Source: CAD feature listing. Evaluate the final solid. Frame: model axes, mm. A direction names the side the tool comes from. Give positions to 0.01 mm unless a question says otherwise; leave off trailing zeros. Loops run counter-clockwise (first coordinate to the right, second up) from the corner with the lowest first, then second, coordinate; pieces in that order, holes last. Notation, with made-up numbers: (6.25, 47.5) -> (42.25, 47.5) arc R13 ccw to (42.25, 60.5) -> close; hole circle Ø4 at (75, 77.25). An arc over 180 degrees is marked (long way). Return JSON: item names as keys, results as strings. Group by question number.
(1) Cut plane C-C on y = 15. Return loops of the section in (x, z).
(2) Pin query (flat end, axial travel): pin 1 (8 mm diameter, centred on x = -1, y = 1.5, fed in from +Z); pin 2 (1.5 mm diameter, centred on x = -6, y = 11.5, fed in from +Z); pin 3 (9 mm diameter, centred on x = 0, y = 0, fed in from -Z); pin 4 (3 mm diameter, centred on x = -1.5, z = 13.5, fed in from -Y). Return the tip coordinate at first contact, or that it passes through.
(3) Draft query along X for faces 4 (the face through (18, 0, 6)), 5 (the face through (-7, -15.429, 5)), 6 (the face through (0, 12.363, 13)). Return one class per face: released by +X, released by -X, zero draft, split by the parting line, or undercut.
(4) Cut plane B-B on z = 4. Give the number of separate pieces and of enclosed holes in the cut face, then the cut area to 3 significant figures.
(5) Cut plane A-A on z = 8.75. Return loops of the section in (x, y).
(6) Cut plane D-D on x = 11. Return loops of the section in (y, z), then the cut area to 3 significant figures.
(7) Access query for faces 1 (the face through (-7, -10.629, 5)), 2 (the face through (-12.363, 0, 13)), 3 (the face through (12.363, 0, 13)). Directions: +Z, -Z, +X, -X, +Y, -Y. A direction counts if a zero-diameter tool reaches every point of the face in a straight line with its end or side. Return the directions, or none.
(8) Ray query, line 1 (Y direction, x = 0, z = 12.3); line 2 (Y direction, x = -10, z = 4.75); line 3 (Z direction, x = -13, y = -13.5). Return the intervals inside material, ascending. Write a range as from..to.
```python
from build123d import *

# Parameters (mm, degrees)
BOSS_EXTRUDE1_DEPTH = 11.868131868
SKETCH2_R           = 1.5
CUT_EXTRUDE1_DEPTH  = 5
BOSS_EXTRUDE2_DEPTH = 2.769230769
SKETCH7_W           = 8.5
SKETCH7_H           = 4.8
SKETCH7_W_2         = 0.5
SKETCH7_H_2         = 0.5
CUT_EXTRUDE2_DEPTH  = 10


with BuildPart() as part:
    # Sketch1 → Boss-Extrude1 (new body)
    with BuildSketch(Plane.XY):
        with BuildLine():
            Line((-16, 18), (16, 18))
            ThreePointArc((16, 18), (17.414213562, 17.414213562), (18, 16))
            Line((18, 16), (18, -16))
            ThreePointArc((18, -16), (17.414213562, -17.414213562), (16, -18))
            Line((16, -18), (-16, -18))
            ThreePointArc((-16, -18), (-17.414213562, -17.414213562), (-18, -16))
            Line((-18, -16), (-18, 16))
            ThreePointArc((-18, 16), (-17.414213562, 17.414213562), (-16, 18))
        make_face()
    extrude(amount=BOSS_EXTRUDE1_DEPTH)

    # Sketch2 → Cut-Extrude1 (cut)
    with BuildSketch(Plane(origin=(0, 0, 0), x_dir=(-1, 0, 0), z_dir=(0, 0, -1))):
        with Locations((-13.554503907, -13.802086098)):
            Circle(SKETCH2_R)
        with Locations((14.445496093, 14.197913902)):
            Circle(SKETCH2_R)
    extrude(amount=-CUT_EXTRUDE1_DEPTH, mode=Mode.SUBTRACT)

    # Sketch3 → Boss-Extrude2 (add)
    with BuildSketch(Plane.XY.offset(11.868131868)):
        with BuildLine():
            Line((-10.362637363, 12.362637363), (10.362637363, 12.362637363))
            ThreePointArc((10.362637363, 12.362637363), (11.776850925, 11.776850925), (12.362637363, 10.362637363))
            Line((12.362637363, 10.362637363), (12.362637363, -10.362637363))
            ThreePointArc((12.362637363, -10.362637363), (11.776850925, -11.776850925), (10.362637363, -12.362637363))
            Line((10.362637363, -12.362637363), (-10.362637363, -12.362637363))
            ThreePointArc((-10.362637363, -12.362637363), (-11.776850925, -11.776850925), (-12.362637363, -10.362637363))
            Line((-12.362637363, -10.362637363), (-12.362637363, 10.362637363))
            ThreePointArc((-12.362637363, 10.362637363), (-11.776850925, 11.776850925), (-10.362637363, 12.362637363))
        make_face()
    extrude(amount=BOSS_EXTRUDE2_DEPTH)

    # Sketch4 → Revolve1 (revolve)
    with BuildSketch(Plane(origin=(0, 0, 0), x_dir=(1, 0, 0), z_dir=(0, 1, 0)), mode=Mode.PRIVATE) as revolve1_sk:
        Polygon((-8.33139296, -14.637362637), (-8.202720326, -14.837362637), (-8.040760547, -14.837362637), (-7.912087912, -14.637362637), align=None)
    revolve(revolve1_sk.sketch.rotate(Axis((0, 0, 15.476177455), (0, 0, 1)), 180), axis=Axis((0, 0, 15.476177455), (0, 0, 1)))

    # Sketch5 → Cut-Revolve1 (revolve, cut)
    with BuildSketch(Plane(origin=(0, 0, 0), x_dir=(1, 0, 0), z_dir=(0, 1, 0)), mode=Mode.PRIVATE) as cut_revolve1_sk:
        Polygon((-7.912087912, -14.637362637), (-5.918480504, -13.782101407), (-5.718480504, -13.782101407), (-5.718480504, -13.582101407), (-5.518480504, -13.582101407), (-5.518480504, -13.382101407), (-5.318480504, -13.382101407), (-5.318480504, -13.182101407), (-5.118480504, -13.182101407), (-5.118480504, -12.982101407), (-4.918480504, -12.982101407), (-4.918480504, -12.782101407), (-4.718480504, -12.782101407), (-4.718480504, -12.582101407), (-4.518480504, -12.582101407), (-4.518480504, -12.382101407), (-4.318480504, -12.382101407), (-4.318480504, -12.182101407), (-4.118480504, -12.182101407), (-4.118480504, -11.982101407), (-3.918480504, -11.982101407), (-3.918480504, -11.782101407), (0, -11.782101407), (0, -14.637362637), align=None)
    revolve(cut_revolve1_sk.sketch.rotate(Axis((0, 0, 19.146341311), (0, 0, -1)), 180), axis=Axis((0, 0, 19.146341311), (0, 0, -1)), mode=Mode.SUBTRACT)

    # Sketch6 → Revolve2 (revolve)
    with BuildSketch(Plane(origin=(0, 0, 0), x_dir=(1, 0, 0), z_dir=(0, 1, 0))):
        with BuildLine():
            Line((-3.308329692, -11.782101407), (-3.308329692, -12.908378043))
            Line((-3.308329692, -12.908378043), (-2.963068503, -12.908378043))
            ThreePointArc((-2.963068503, -12.908378043), (-1.670669607, -14.043416814), (0, -14.452649))
            Line((0, -14.452649), (0, -11.782101407))
            Line((0, -11.782101407), (-3.308329692, -11.782101407))
        make_face()
    revolve(axis=Axis((0, 0, 14.452649), (0, 0, -1)))

    # Sketch7 → Cut-Extrude2 (cut)
    with BuildSketch(Plane(origin=(0, 0, 0), x_dir=(-1, 0, 0), z_dir=(0, 0, -1))):
        with Locations((6.826923077, -13.028571429)):
            Rectangle(SKETCH7_W, SKETCH7_H)
        with Locations((4.064707138, -12.284956035)):
            Rectangle(SKETCH7_W_2, SKETCH7_H_2, mode=Mode.SUBTRACT)
        with Locations((5.906184431, -12.284956035)):
            Rectangle(SKETCH7_W_2, SKETCH7_H_2, mode=Mode.SUBTRACT)
        with Locations((7.747661723, -12.284956035)):
            Rectangle(SKETCH7_W_2, SKETCH7_H_2, mode=Mode.SUBTRACT)
        with Locations((9.589139016, -12.284956035)):
            Rectangle(SKETCH7_W_2, SKETCH7_H_2, mode=Mode.SUBTRACT)
    extrude(amount=-CUT_EXTRUDE2_DEPTH, mode=Mode.SUBTRACT)


solid = part.part
```
Answers:
{
 "1": {"outline": "(-18, 0) -> (-15.71, 0) -> (-15.71, 5) -> (-13.18, 5) -> (-13.18, 0) -> (18, 0) -> (18, 11.87) -> (-18, 11.87) -> close"},
 "2": {"pin 1": "z = 14.45", "pin 2": "z = 14.64", "pin 3": "z = 0", "pin 4": "y = -12.36"},
 "3": {"face 4": "released by +X", "face 5": "undercut", "face 6": "zero draft"},
 "4": {"separate pieces": "5", "enclosed holes": "3", "area": "1,240 mm²"},
 "5": {"outline": "(-18, -16) arc R2 ccw to (-16, -18) -> (16, -18) arc R2 ccw to (18, -16) -> (18, 16) arc R2 ccw to (16, 18) -> (-16, 18) arc R2 ccw to (-18, 16) -> close; (-9.84, -12.53) -> (-9.34, -12.53) -> (-9.34, -12.03) -> (-9.84, -12.03) -> close; (-8, -12.53) -> (-7.5, -12.53) -> (-7.5, -12.03) -> (-8, -12.03) -> close; (-6.16, -12.53) -> (-5.66, -12.53) -> (-5.66, -12.03) -> (-6.16, -12.03) -> close; (-4.31, -12.53) -> (-3.81, -12.53) -> (-3.81, -12.03) -> (-4.31, -12.03) -> close; hole (-11.08, -15.43) -> (-2.58, -15.43) -> (-2.58, -10.63) -> (-11.08, -10.63) -> close"},
 "6": {"outline": "(-18, 0) -> (18, 0) -> (18, 11.87) -> (12.26, 11.87) -> (12.26, 14.64) -> (-12.26, 14.64) -> (-12.26, 11.87) -> (-18, 11.87) -> close", "area": "495 mm²"},
 "7": {"face 1": "-Z", "face 2": "+Z, -X, +Y, -Y", "face 3": "+Z, +X, +Y, -Y"},
 "8": {"line 1": "-12.36..-4.32, -3.31..3.31, 4.32..12.36", "line 2": "-18..-15.43, -10.63..18", "line 3": "0..11.87"}
}
